Could you check a few things on this model? Use its own coordinates, in mm. Face numbers are marked on the shaded views. A direction names the side the tool comes from. Coordinates: 2 decimals unless noted, no trailing zeros. Order: outer loops, then holes, each group sorted by start corner. A loop starts at its lowest first (then second) coordinate and runs counter-clockwise, first axis right, second up. Notation, with made-up numbers: (14.5, 82.25) - (34.5, 82.25) arc R23 ccw to (34.5, 112.25) - close; hole circle Ø6 at (13, 49). An arc over 180 degrees is marked (long way). Answer as a JSON object with one key per item and string values. Group by question number.
(1) Imagine slicing it at C-C, the plane y = -1.4. Write out the boundary of the cut face in (x, z).
(2) Imagine slicing it at B-B, the plane x = 5. Write out the boundary of the cut face in (y, z).
(3) Imagine slicing it at A-A, the plane z = -17. Write out the boundary of the cut face in (x, y).
(4) We'd pull the mould along Z, two halves only. Please class the marked faces 1 and 2: pulls with the +Z half, pulls with the -Z half, needs draft (parallel to the pull), parting line crosses it, or undercut.
(5) Please list where these lines run through material, in increasing order: probe 1 along Y at (x, z) = (-2, 10); probe 2 along Y at (x, z) = (-7.5, 28.5); probe 3 along X at (y, z) = (-3.5, 3.5).
(6) Will these pins go through, and if not, where does the flat tip stop? P1, Ø1, axis at x = -20, y = -2.5, coming from the -Z side; P2, Ø0.5, axis at x = -0.5, y = -3.5, coming from the +Z side; P3, Ø1, axis at x = 2.5, z = 29.5, coming from the -Y side.
(7) Which directions (+Z, -Z, +X, -X, +Y, -Y) give clear straight access to the entire face, cutting with the end or side of a thin tool? Please do the marked faces 3 and 4.
(8) Imagine slicing it at D-D, the plane z = 14. Write out the boundary of the cut face in (x, y).
from build123d import *

# Parameters (mm, degrees)
F1_DEPTH = 3
F2_R     = 27.42995
F3_DEPTH = 1
F5_W     = 2.706106
F5_H     = 85.87949
F6_DEPTH = 1


with BuildPart() as f1:
    # F0 (on Front) → F1 (new body)
    with BuildSketch(Plane.XZ):
        Polygon((0, 56.272782), (-47.566082, -28.044742), (49.765669, -28.044742), align=None)
    extrude(amount=F1_DEPTH)

    # F2 (on face) → F3 (cut)
    with BuildSketch(Plane.XZ.offset(3)):
        Circle(F2_R)
    extrude(amount=-F3_DEPTH, mode=Mode.SUBTRACT)

    # F5 (on face) → F6 (join)
    with BuildSketch(Plane.XZ.offset(3)):
        with Locations((0, 12.268752)):
            Rectangle(F5_W, F5_H)
    extrude(amount=F6_DEPTH)


solid = f1.part
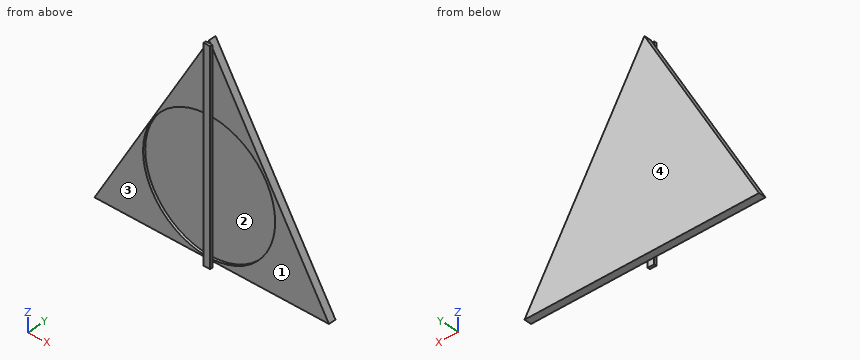
Result set:
{
 "1": {"outline": "(-47.57, -28.04) - (49.77, -28.04) - (0, 56.27) - close"},
 "2": {"outline": "(-3, -28.04) - (0, -28.04) - (0, 47.8) - (-3, 47.8) - (-3, 26.97) - (-2, 26.97) - (-2, -26.97) - (-3, -26.97) - close"},
 "3": {"outline": "(-41.34, -3) - (-21.53, -3) - (-21.53, -2) - (21.53, -2) - (21.53, -3) - (43.25, -3) - (43.25, 0) - (-41.34, 0) - close; (-1.35, -4) - (1.35, -4) - (1.35, -3) - (-1.35, -3) - close"},
 "4": {"face 1": "needs draft", "face 2": "undercut"},
 "5": {"probe 1": "y = -2 to 0", "probe 2": "y = -3 to 0", "probe 3": "x = -1.35 to 1.35"},
 "6": {"P1": "stops at z = -28.04", "P2": "stops at z = 55.21", "P3": "stops at y = -3"},
 "7": {"face 3": "+Z, -Z, -X, -Y", "face 4": "+Z, -Z, +X, -X, +Y"},
 "8": {"outline": "(-23.85, -3) - (-23.59, -3) - (-23.59, -2) - (23.59, -2) - (23.59, -3) - (24.95, -3) - (24.95, 0) - (-23.85, 0) - close; (-1.35, -4) - (1.35, -4) - (1.35, -3) - (-1.35, -3) - close"}
}
